```python
from build123d import *

# Parameters (mm, degrees)
ESQUISSE1_R          = 3.5
ESQUISSE1_R_2        = 1.5
BOSS_EXTRU_2_DEPTH   = 2.5
BOSS_EXTRU_2_2_DEPTH = 2.5
BOSS_EXTRU_2_3_DEPTH = 2.5
BOSS_EXTRU_2_4_DEPTH = 2.5
BOSS_EXTRU_3_DEPTH   = 1


with BuildPart() as part:
    # Esquisse1 → Boss.-Extru.2 (new body)
    with BuildSketch(Plane.XY):
        with Locations((-24.5, 29)):
            Circle(ESQUISSE1_R)
        with Locations((-24.5, 29)):
            Circle(ESQUISSE1_R_2, mode=Mode.SUBTRACT)
    extrude(amount=BOSS_EXTRU_2_DEPTH)



with BuildPart() as body_2:
    # Esquisse1 → Boss.-Extru.2 2 (new body)
    with BuildSketch(Plane.XY):
        with Locations((24.5, 29)):
            Circle(ESQUISSE1_R)
        with Locations((24.5, 29)):
            Circle(ESQUISSE1_R_2, mode=Mode.SUBTRACT)
    extrude(amount=BOSS_EXTRU_2_2_DEPTH)


with BuildPart() as body_3:
    # Esquisse1 → Boss.-Extru.2 3 (new body)
    with BuildSketch(Plane.XY):
        with Locations((-24.5, -29)):
            Circle(ESQUISSE1_R)
        with Locations((-24.5, -29)):
            Circle(ESQUISSE1_R_2, mode=Mode.SUBTRACT)
    extrude(amount=BOSS_EXTRU_2_3_DEPTH)


with BuildPart() as body_4:
    # Esquisse1 → Boss.-Extru.2 4 (new body)
    with BuildSketch(Plane.XY):
        with Locations((24.5, -29)):
            Circle(ESQUISSE1_R)
        with Locations((24.5, -29)):
            Circle(ESQUISSE1_R_2, mode=Mode.SUBTRACT)
    extrude(amount=BOSS_EXTRU_2_4_DEPTH)


with BuildPart() as part_1:
    add(part.part)

    add(body_2.part)  # Boss.-Extru.3 merges body 2

    add(body_3.part)  # Boss.-Extru.3 merges body 3

    add(body_4.part)  # Boss.-Extru.3 merges body 4
    # Esquisse3 → Boss.-Extru.3 (add)
    with BuildSketch(Plane.XY.offset(2.5)):
        Polygon((24.5, 27.5), (24.5, -27.5), (-24.5, -27.5), (-24.5, 27.5), (-22.5, 27.5), (-22.5, -25.5), (22.5, -25.5), (22.5, 27.5), align=None)
    extrude(amount=-BOSS_EXTRU_3_DEPTH)


solid = part_1.part
```
The model under review builds one solid part; all positions refer to its coordinate system, in mm. A direction names the side the tool comes from. Give positions to 0.01 mm unless a question says otherwise; leave off trailing zeros. Write each loop counter-clockwise with the first axis right and the second up, starting at its lowest first coordinate (ties: lowest second). Pieces come first, ordered by that corner, then holes. Notation, with made-up numbers: (27.5, 53) -> (84.5, 53) arc R25 cw to (84.5, 78) -> close; hole circle Ø9 at (-10, 30). An arc over 180 degrees is marked (long way). Put each result on its own line as item: value.
(1) Tool access review of faces 3 (the flat face through (0, -26, 2.5)), 4 (the flat face through (0, -26, 1.5)): name each direction out of +Z, -Z, +X, -X, +Y, -Y from which nothing blocks a thin tool from reaching the whole face with its end or side.
Results are:
face 3: +Z, +X, -X, +Y, -Y
face 4: -Z
(2) We need section A-A, the plane y = 29. Give the boundary of the cut face in (x, z), and give its area (3 significant figures).
Results are:
outline: (-28, 0) -> (-26, 0) -> (-26, 2.5) -> (-28, 2.5) -> close; (-23, 0) -> (-21, 0) -> (-21, 2.5) -> (-23, 2.5) -> close; (21, 0) -> (23, 0) -> (23, 2.5) -> (21, 2.5) -> close; (26, 0) -> (28, 0) -> (28, 2.5) -> (26, 2.5) -> close
area: 20.0 mm²
(3) We need section D-D, the plane y = -26.5. Give the boundary of the cut face in (x, z), and give its area (3 significant figures).
Results are:
outline: (-26.95, 0) -> (-22.05, 0) -> (-22.05, 1.5) -> (22.05, 1.5) -> (22.05, 0) -> (26.95, 0) -> (26.95, 2.5) -> (-26.95, 2.5) -> close
area: 68.6 mm²
(4) We need section C-C, the plane y = -15. Give the boundary of the cut face in (x, z), and give its area (3 significant figures).
Results are:
outline: (-24.5, 1.5) -> (-22.5, 1.5) -> (-22.5, 2.5) -> (-24.5, 2.5) -> close; (22.5, 1.5) -> (24.5, 1.5) -> (24.5, 2.5) -> (22.5, 2.5) -> close
area: 4.00 mm²
(5) The part is to be moulded in two halves that separate along Y. For faces 1 (the cylindrical face through (-27.3, -31.1, 1.2)), 2 (the flat face through (-25, -31, 0)), say which applies: pulls with the +Y half, pulls with the -Y half, needs draft (parallel to the pull), parting line crosses it, or undercut.
Results are:
face 1: undercut
face 2: needs draft
(6) We need section B-B, the plane z = 0.55. Give the boundary of the cut face in (x, y).
Results are:
outline: circle Ø7 at (-24.5, -29); circle Ø7 at (-24.5, 29); circle Ø7 at (24.5, -29); circle Ø7 at (24.5, 29); hole circle Ø3 at (-24.5, -29); hole circle Ø3 at (-24.5, 29); hole circle Ø3 at (24.5, -29); hole circle Ø3 at (24.5, 29)
(7) To check wall thickness, follow probe 1 along Y at (x, z) = (-24.5, 1.2); probe 2 along X at (y, z) = (29, 0.65); probe 3 along X at (y, z) = (15.5, 2.15). State the ranges of each line that lie inside material, in increasing order. Write a range as from..to.
Results are:
probe 1: -32.5..-30.5, -27.5..-25.5, 25.5..27.5, 30.5..32.5
probe 2: -28..-26, -23..-21, 21..23, 26..28
probe 3: -24.5..-22.5, 22.5..24.5
(8) For pin 1 Ø0.5 at (x, z) = (10.5, 2) entering from +Y; pin 2 Ø0.8 at (y, z) = (-12.5, 2) entering from +X; pin 3 Ø1.1 at (x, z) = (3.5, 2) entering from -Y, all flat-tipped, find the tip position at first contact; note any pin that passes through.
Results are:
pin 1: y = -25.5
pin 2: x = 24.5
pin 3: y = -27.5
